The listing builds one solid part. Answer for the finished solid, in the listing's coordinates (mm). A direction names the side the tool comes from. Round coordinates to 2 decimals unless told otherwise and drop trailing zeros. Loops run counter-clockwise (first coordinate to the right, second up) from the corner with the lowest first, then second, coordinate; pieces in that order, holes last. Notation, with made-up numbers: M 47,-5 L 85,-5 A19 cw 85,4 Z; hole C -27.5,82.25 d11. An arc over 180 degrees is marked long. Put each result on its own line as item: value. Start each with the question number.
(1) Which of the six approach directions +Z, -Z, +X, -X, +Y, -Y give full straight-line access (tool end or side, diameter ignored) to faces 1 (the face through (-0.3, -0.5, -10.5)), 2 (the face through (-0.17, 0.5, 6.27)), 3 (the face through (-12, -0.2, 7.5))?
(2) Section A-A, the plane z = -4 is taken. Determine the outline of the cut face in (x, y).
(3) Determine the mould class of faces 4 (the face through (12, -0.2, 7.5)), 5 (the face through (18.4, -0.5, 4.5)), 6 (the face through (-25, -0.5, -2.9)), 7 (the face through (-17.499, -0.493, -1.615)) for opening direction X: released by +X, released by -X, zero draft, split by the parting line, or undercut.
(4) Section B-B, the plane x = -18.25 is taken. Determine the outline of the cut face in (y, z).
(5) Section C-C, the plane x = -9 is taken. Determine the outline of the cut face in (y, z).
(6) Flat-ended cylindrical pins translate along their axes: P1, Ø1.5, axis at y = 2.5, z = 8, coming from the -X side; P2, Ø6, axis at x = 8.5, z = 0.5, coming from the +Y side; P3, Ø0.5, axis at x = -20, y = -0.5, coming from the +Z side; P4, Ø3, axis at x = 18.25, z = -4, coming from the +Y side. Find the tip coordinate at first contact, or state that the pin passes through.
(7) Straight lines are drawn through the part: line 1 (X direction, y = -0.8, z = -4); line 2 (Z direction, x = 7, y = 1.5); line 3 (Y direction, x = 14, z = -3.5). For each, find the intervals that lie inside material, in ascending order.
(8) Section D-D, the plane z = -0.5 is taken. Determine the outline of the cut face in (x, y), then the cut area to 3 significant figures.
```python
from build123d import *

# Parameters (mm, degrees)
SKETCH2_W               = 50
SKETCH2_H               = 21
BASE_FLANGE1_DEPTH      = 1
HEM1_START              = -25
HEM1_DEPTH              = 50
HEM1_2_DEPTH            = 50
CUT_EXTRUDE1_DEPTH      = 28.408940147
CUT_EXTRUDE1_DEPTH_BACK = 28.408940147
SKETCH5_W               = 13
SKETCH5_H               = 6
SKETCH6_R               = 2.5
CUT_EXTRUDE2_DEPTH      = 28.408940147


# Read off the part's stored shape, not the designer's step: Hem1
# Sheet-metal steps are written as plain solids
with BuildPart() as part:
    # Sketch2 → Base-Flange1 (new body)
    with BuildSketch(Plane(origin=(0, 0, 0), x_dir=(1, 0, 0), z_dir=(0, 1, 0))):
        Rectangle(SKETCH2_W, SKETCH2_H)
    extrude(amount=-BASE_FLANGE1_DEPTH)

    # Hem1 outline → Hem1 (cut)
    with BuildSketch(Plane.YZ.offset(HEM1_START)):
        with BuildLine():
            ThreePointArc((-1, 8), (-0.736067978, 9.118033989), (0, 10))
            Line((0, 10), (0, 10.5))
            Line((0, 10.5), (-1, 10.5))
            Line((-1, 10.5), (-1, 8))
        make_face()
    extrude(amount=HEM1_DEPTH, mode=Mode.SUBTRACT)

    # Hem1 2 outline → Hem1 2 (add)
    with BuildSketch(Plane.YZ.offset(HEM1_START)):
        with BuildLine():
            Line((0.75, 6.700961894), (0.25, 5.834936491))
            ThreePointArc((0.25, 5.834936491), (3.995508667, 8.149788152), (0, 10))
            Line((0, 10), (0, 8))
            ThreePointArc((0, 8), (2.799038106, 8.75), (0.75, 6.700961894))
        make_face()
    extrude(amount=HEM1_2_DEPTH)

    # Sketch5 → Cut-Extrude1 (cut, two sides: drawn at the far end of the back side and taken through both)
    with BuildSketch(Plane(origin=(0, 0, 0), x_dir=(1, 0, 0), z_dir=(0, 1, 0)).offset(-CUT_EXTRUDE1_DEPTH_BACK)):
        with Locations((18.5, -7.5)):
            Rectangle(SKETCH5_W, SKETCH5_H)
        with Locations((-18.5, -7.5)):
            Rectangle(SKETCH5_W, SKETCH5_H)
    extrude(amount=CUT_EXTRUDE1_DEPTH + CUT_EXTRUDE1_DEPTH_BACK, mode=Mode.SUBTRACT)

    # Sketch6 → Cut-Extrude2 (cut, through all)
    with BuildSketch(Plane(origin=(0, 0, 0), x_dir=(1, 0, 0), z_dir=(0, 1, 0))):
        with Locations(Location((18.25, 4, 0), (0, 0, 270))):
            Circle(SKETCH6_R)
        with Locations(Location((-18.25, 4, 0), (0, 0, 270))):
            Circle(SKETCH6_R)
    extrude(amount=-CUT_EXTRUDE2_DEPTH, mode=Mode.SUBTRACT)


solid = part.part
```
Recorded:
1. face 1: -Z, +X, -X, +Y, -Y
1. face 2: +X, -X
1. face 3: +Z, -X, +Y, -Y
2. outline: M -25,-1 L -20.75,-1 L -20.75,0 L -25,0 Z; M -15.75,-1 L 15.75,-1 L 15.75,0 L -15.75,0 Z; M 20.75,-1 L 25,-1 L 25,0 L 20.75,0 Z
3. face 4: released by +X
3. face 5: zero draft
3. face 6: released by -X
3. face 7: undercut
4. outline: M -1,-10.5 L 0,-10.5 L 0,-6.5 L -1,-6.5 Z; M -1,-1.5 L 0,-1.5 L 0,4.5 L -1,4.5 Z
5. outline: M -1,-10.5 L 0,-10.5 L 0,8 A1.5 cw long 0.75,6.7 L 0.25,5.83 A2.5 ccw long -1,8 Z
6. P1: stops at x = -12
6. P2: stops at y = 0
6. P3: stops at z = 4.5
6. P4: passes through
7. line 1: x = -25 to -20.75, -15.75 to 15.75, 20.75 to 25
7. line 2: z = 5.5 to 6.5, 9.5 to 10.5
7. line 3: y = -1 to 0
8. outline: M -25,-1 L 25,-1 L 25,0 L -25,0 Z
8. area: 50.0 mm²
